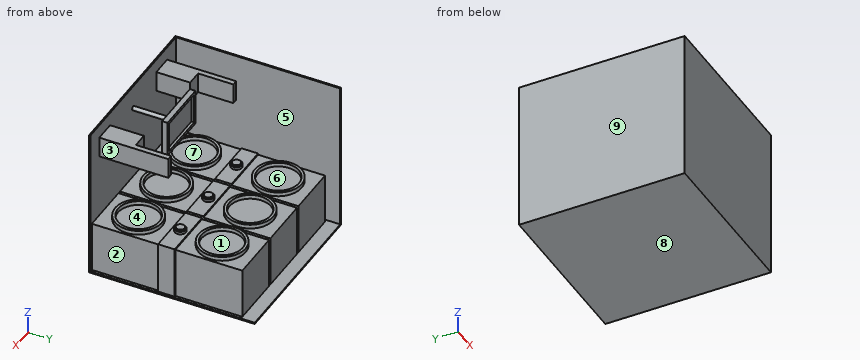
from build123d import *

# Parameters (mm, degrees)
SKETCH_1_W           = 120
SKETCH_1_H           = 110
EXTRUDE_1_DEPTH      = 120
SKETCH_2_W           = 119
SKETCH_2_H           = 119
CUT_EXTRUDE_1_DEPTH  = 109
SKETCH_54_W          = 37
SKETCH_54_H          = 37
EXTRUDE_32_DEPTH     = 109
SKETCH_55_W          = 37
SKETCH_55_H          = 12
EXTRUDE_33_DEPTH     = 1
SKETCH_56_R          = 4
EXTRUDE_34_DEPTH     = 2
SKETCH_57_R          = 3
EXTRUDE_35_DEPTH     = 1
SKETCH_59_R          = 17
SKETCH_59_R_2        = 15
EXTRUDE_36_DEPTH     = 3
SKETCH_60_W          = 38
SKETCH_60_H          = 12
EXTRUDE_37_DEPTH     = 1
SKETCH_61_R          = 1.5
EXTRUDE_38_DEPTH     = 31
SKETCH_62_W          = 38.68188347
SKETCH_62_H          = 26.17234464
EXTRUDE_39_DEPTH     = 4
SKETCH_63_W          = 35.246239362
SKETCH_63_H          = 21.9665941
CUT_EXTRUDE_9_DEPTH  = 2
SKETCH_65_W          = 15
SKETCH_65_H          = 15
EXTRUDE_40_DEPTH     = 50
SKETCH_66_W          = 11.082023192
SKETCH_66_H          = 25.508987467
CUT_EXTRUDE_10_DEPTH = 30


with BuildPart() as part:
    # 스케치1 → 보스-돌출1 (new body)
    with BuildSketch(Plane(origin=(0, 0, 0), x_dir=(1, 0, 0), z_dir=(0, 1, 0))):
        Rectangle(SKETCH_1_W, SKETCH_1_H)
    extrude(amount=EXTRUDE_1_DEPTH)

    # 스케치2 → 컷-돌출1 (cut)
    with BuildSketch(Plane.XY.offset(55)):
        with Locations((0.5, 60.5)):
            Rectangle(SKETCH_2_W, SKETCH_2_H)
    extrude(amount=-CUT_EXTRUDE_1_DEPTH, mode=Mode.SUBTRACT)

    # 스케치54 → 보스-돌출32 (add)
    with BuildSketch(Plane(origin=(0, 1, 0), x_dir=(1, 0, 0), z_dir=(0, 1, 0))):
        with Locations((-38.5, 35.5)):
            Rectangle(SKETCH_54_W, SKETCH_54_H)
        with Locations((0.5, 35.5)):
            Rectangle(SKETCH_54_W, SKETCH_54_H)
        with Locations((39.5, 35.5)):
            Rectangle(SKETCH_54_W, SKETCH_54_H)
    extrude(amount=EXTRUDE_32_DEPTH)

    # 스케치55 → 보스-돌출33 (add)
    with BuildSketch(Plane.XY.offset(-17)):
        with Locations((-38.5, 55.5)):
            Rectangle(SKETCH_55_W, SKETCH_55_H)
        with Locations((0.5, 55.5)):
            Rectangle(SKETCH_55_W, SKETCH_55_H)
        with Locations((39.5, 55.5)):
            Rectangle(SKETCH_55_W, SKETCH_55_H)
    extrude(amount=EXTRUDE_33_DEPTH)

    # 스케치56 → 보스-돌출34 (add)
    with BuildSketch(Plane.XY.offset(-16)):
        with Locations((-38.5, 55.5)):
            Circle(SKETCH_56_R)
        with Locations(Location((39.5, 55.5, 0), (0, 0, 180))):
            Circle(SKETCH_56_R)
        with Locations((0.5, 55.5)):
            Circle(SKETCH_56_R)
    extrude(amount=EXTRUDE_34_DEPTH)

    # 스케치57 → 보스-돌출35 (add)
    with BuildSketch(Plane.XY.offset(-14)):
        with Locations((0.5, 55.5)):
            Circle(SKETCH_57_R)
        with Locations((39.5, 55.5)):
            Circle(SKETCH_57_R)
        with Locations((-38.5, 55.5)):
            Circle(SKETCH_57_R)
    extrude(amount=EXTRUDE_35_DEPTH)

    # 스케치59 → 보스-돌출36 (add)
    # profile 1 of 6: a face of its own
    with BuildSketch(Plane.XY.offset(-17)):
        with Locations(Location((-38.5, 25.25, 0), (0, 0, 180))):
            Circle(SKETCH_59_R)
        with Locations((-38.5, 25.25)):
            Circle(SKETCH_59_R_2, mode=Mode.SUBTRACT)
    # profile 2 of 6: a face of its own
    with BuildSketch(Plane.XY.offset(-17)):
        with Locations(Location((39.5, 25.25, 0), (0, 0, 180))):
            Circle(SKETCH_59_R)
        with Locations(Location((39.5, 25.25, 0), (0, 0, 180))):
            Circle(SKETCH_59_R_2, mode=Mode.SUBTRACT)
    # profile 3 of 6: a face of its own
    with BuildSketch(Plane.XY.offset(-17)):
        with Locations(Location((39.5, 85.75, 0), (0, 0, 180))):
            Circle(SKETCH_59_R)
        with Locations((39.5, 85.75)):
            Circle(SKETCH_59_R_2, mode=Mode.SUBTRACT)
    # profile 4 of 6: a face of its own
    with BuildSketch(Plane.XY.offset(-17)):
        with Locations(Location((-38.5, 85.75, 0), (0, 0, 180))):
            Circle(SKETCH_59_R)
        with Locations(Location((-38.5, 85.75, 0), (0, 0, 180))):
            Circle(SKETCH_59_R_2, mode=Mode.SUBTRACT)
    # profile 5 of 6: a face of its own
    with BuildSketch(Plane.XY.offset(-17)):
        with Locations(Location((0.5, 25.25, 0), (0, 0, 180))):
            Circle(SKETCH_59_R)
        with Locations((0.5, 25.25)):
            Circle(SKETCH_59_R_2, mode=Mode.SUBTRACT)
    # profile 6 of 6: a face of its own
    with BuildSketch(Plane.XY.offset(-17)):
        with Locations(Location((0.5, 85.75, 0), (0, 0, 180))):
            Circle(SKETCH_59_R)
        with Locations(Location((0.5, 85.75, 0), (0, 0, 180))):
            Circle(SKETCH_59_R_2, mode=Mode.SUBTRACT)
    extrude(amount=EXTRUDE_36_DEPTH)

    # 스케치60 → 보스-돌출37 (add)
    with BuildSketch(Plane(origin=(58, 0, 0), x_dir=(0, 0, -1), z_dir=(1, 0, 0))):
        with Locations((35, 55.5)):
            Rectangle(SKETCH_60_W, SKETCH_60_H)
    extrude(amount=EXTRUDE_37_DEPTH)

    # 스케치61 → 보스-돌출38 (add)
    with BuildSketch(Plane(origin=(0, 1, 0), x_dir=(1, 0, 0), z_dir=(0, 1, 0))):
        with Locations((0.5, -37.648978871)):
            Circle(SKETCH_61_R)
    extrude(amount=EXTRUDE_38_DEPTH)

    # 스케치62 → 보스-돌출39 (add)
    with BuildSketch(Plane(origin=(0, 32, 0), x_dir=(1, 0, 0), z_dir=(0, 1, 0))):
        with Locations((0.5, -37.648978871)):
            Rectangle(SKETCH_62_W, SKETCH_62_H)
    extrude(amount=EXTRUDE_39_DEPTH)

    # 스케치63 → 컷-돌출9 (cut)
    with BuildSketch(Plane(origin=(0, 36, 0), x_dir=(1, 0, 0), z_dir=(0, 1, 0))):
        with Locations((0.5, -37.642682595)):
            Rectangle(SKETCH_63_W, SKETCH_63_H)
    extrude(amount=-CUT_EXTRUDE_9_DEPTH, mode=Mode.SUBTRACT)

    # 스케치65 → 보스-돌출40 (add)
    with BuildSketch(Plane(origin=(0, 1, 0), x_dir=(1, 0, 0), z_dir=(0, 1, 0))):
        with Locations((-39.153156526, -37.716582515)):
            Rectangle(SKETCH_65_W, SKETCH_65_H)
        with Locations((40.153156526, -37.716582515)):
            Rectangle(SKETCH_65_W, SKETCH_65_H)
    extrude(amount=EXTRUDE_40_DEPTH)

    # 스케치66 → 컷-돌출10 (cut)
    with BuildSketch(Plane.XY.offset(45.216582515)):
        with Locations((-37.194168122, 38.245506267)):
            Rectangle(SKETCH_66_W, SKETCH_66_H)
        with Locations((38.194168122, 38.245506267)):
            Rectangle(SKETCH_66_W, SKETCH_66_H)
    extrude(amount=-CUT_EXTRUDE_10_DEPTH, mode=Mode.SUBTRACT)


solid = part.part
Verification items for the finished model (mm, model axes). Face numbers are marked on the shaded views. A direction names the side the tool comes from. Coordinates: 2 decimals unless noted, no trailing zeros. Order: outer loops, then holes, each group sorted by start corner. A loop starts at its lowest first (then second) coordinate and runs counter-clockwise, first axis right, second up.
1. Sectioned sample at A-A, the plane y = 45. Record the cut outline in (x, z).
Results found:
outline: (-60, -55) - (60, -55) - (60, -54) - (58, -54) - (58, -17) - (21, -17) - (21, -54) - (19, -54) - (19, -17) - (-18, -17) - (-18, -54) - (-20, -54) - (-20, -17) - (-57, -17) - (-57, -54) - (-59, -54) - (-59, 55) - (-60, 55) - close; (-46.65, 30.22) - (-42.74, 30.22) - (-42.74, 45.22) - (-46.65, 45.22) - close; (43.74, 30.22) - (47.65, 30.22) - (47.65, 45.22) - (43.74, 45.22) - close
2. Scan lines: line 1 (X direction, y = 28, z = 45); line 2 (X direction, y = 106, z = -30.5); line 3 (Y direction, x = 0, z = -15). Record each from-to range of solid material in increasing order.
Results found:
line 1: x = -60 to -59, -46.65 to -42.74, 43.74 to 47.65
line 2: x = -60 to -59, -57 to -20, -18 to 19, 21 to 58
line 3: y = 0 to 1, 8.26 to 10.26, 40.24 to 42.24, 51.53 to 59.47, 68.76 to 70.76, 100.74 to 102.74
3. Sectioned sample at B-B, the plane z = -44.5. Record the cut outline in (x, y), and give its area (4 significant figures).
Results found:
outline: (-60, 0) - (60, 0) - (60, 1) - (58, 1) - (58, 49.5) - (59, 49.5) - (59, 61.5) - (58, 61.5) - (58, 110) - (21, 110) - (21, 1) - (19, 1) - (19, 110) - (-18, 110) - (-18, 1) - (-20, 1) - (-20, 110) - (-57, 110) - (-57, 1) - (-59, 1) - (-59, 120) - (-60, 120) - close
area: 12,350 mm2
4. Go/stop test with flat-tipped pins: pin 1 Ø1.5 at (x, z) = (-35.5, 20) entering from -Y; pin 2 Ø4.5 at (x, z) = (-44, 34) entering from +Y; pin 3 Ø16.5 at (y, z) = (35.5, 39) entering from +X; pin 4 Ø8 at (y, z) = (22, -24) entering from +X. Record where each tip stops, or that it passes through.
Results found:
pin 1: stops at y = 0
pin 2: stops at y = 51
pin 3: stops at x = 47.65
pin 4: stops at x = 58
5. Sectioned sample at C-C, the plane x = 52. Record the cut outline in (y, z).
Results found:
outline: (0, -55) - (120, -55) - (120, -54) - (110, -54) - (110, -17) - (97.27, -17) - (97.27, -14) - (94.04, -14) - (94.04, -17) - (77.46, -17) - (77.46, -14) - (74.23, -14) - (74.23, -17) - (61.5, -17) - (61.5, -16) - (49.5, -16) - (49.5, -17) - (36.77, -17) - (36.77, -14) - (33.54, -14) - (33.54, -17) - (16.96, -17) - (16.96, -14) - (13.73, -14) - (13.73, -17) - (1, -17) - (1, 55) - (0, 55) - close
6. Release check for a two-part mould opening along Z. For the marked faces 6, 7, 8 and 9 record: +Z half, -Z half, draft (parallel to the pull), parting line (faces both ways), or undercut.
Results found:
face 6: +Z half
face 7: undercut
face 8: -Z half
face 9: draft
7. Set-up check for the marked faces 1, 2, 3, 4 and 5: record each of +Z, -Z, +X, -X, +Y, -Y from which the full face is reachable in a straight line by a thin tool's end or side.
Results found:
face 1: +Z
face 2: +Z, +X
face 3: +Z, +X, +Y
face 4: none
face 5: +Z, +Y
